The figure shows three views and two pictorial views of one solid part (mm, origin at its lowest corner). Answer the questions. A direction names the side the tool comes from. Coordinates: 2 decimals unless noted, no trailing zeros. Loops run counter-clockwise (first coordinate to the right, second up) from the corner with the lowest first, then second, coordinate; pieces in that order, holes last.
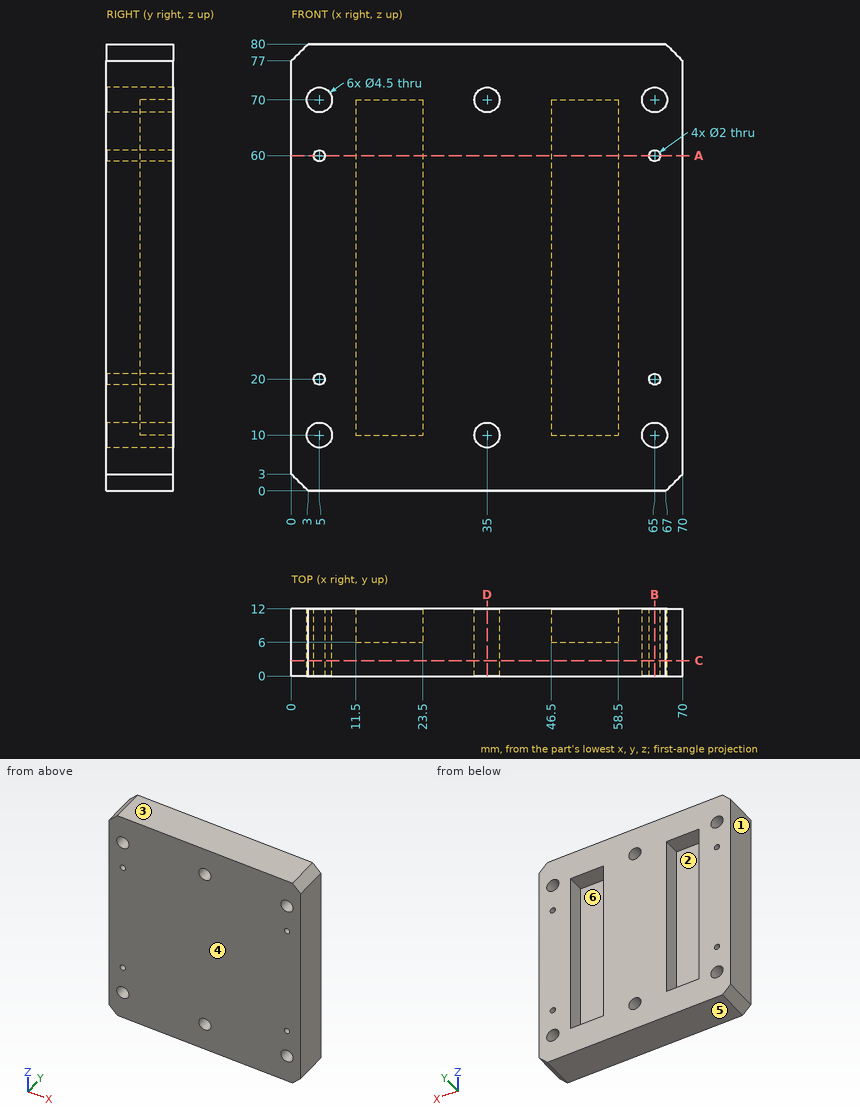
Q1. A cutting plane is placed at B-B (x = 65). Give the vertices of the cut face in (y, z), then the cut area to 3 significant figures.
Findings below:
outline: (0, 0) - (12, 0) - (12, 7.75) - (0, 7.75) - close; (0, 12.25) - (12, 12.25) - (12, 19) - (0, 19) - close; (0, 21) - (12, 21) - (12, 59) - (0, 59) - close; (0, 61) - (12, 61) - (12, 67.75) - (0, 67.75) - close; (0, 72.25) - (12, 72.25) - (12, 80) - (0, 80) - close
area: 804 mm2
Q2. A cutting plane is placed at C-C (y = 2.75). Count the separate pieces of the cut face and the enclosed holes in it, then the cut area to 3 significant figures.
Findings below:
separate pieces: 1
enclosed holes: 10
area: 5,470 mm2
Q3. Which of the six approach directions +Z, -Z, +X, -X, +Y, -Y give full straight-line access (tool end or side, diameter ignored) to the marked faces 1 and 2?
Findings below:
face 1: +Z, -Z, -X, +Y, -Y
face 2: +Y
Q4. Determine the mould class of the marked faces 3, 4, 5 and 6 for opening direction Z: +Z half, -Z half, draft (parallel to the pull), parting line (faces both ways), or undercut.
Findings below:
face 3: +Z half
face 4: draft
face 5: -Z half
face 6: undercut
Q5. A flat-ended cylindrical pin translates along its axis: pin 1 Ø1.5 at (x, z) = (54.5, 63.5) entering from +Y. Find the tip coordinate at first contact, or state that the pin passes through.
Findings below:
pin 1: stops at y = 6
Q6. Straight lines are drawn through the part: probe 1 along X at (y, z) = (11, 52.5); probe 2 along X at (y, z) = (8.25, 20); probe 3 along Z at (x, y) = (19, 9.5). For each, find the intervals that lie inside material, in ascending order.
Findings below:
probe 1: x = 0 to 11.5, 23.5 to 46.5, 58.5 to 70
probe 2: x = 0 to 4, 6 to 11.5, 23.5 to 46.5, 58.5 to 64, 66 to 70
probe 3: z = 0 to 10, 70 to 80
Q7. A cutting plane is placed at A-A (z = 60). Give the vertices of the cut face in (x, y), then the cut area to 3 significant figures.
Findings below:
outline: (0, 0) - (4, 0) - (4, 12) - (0, 12) - close; (6, 0) - (64, 0) - (64, 12) - (58.5, 12) - (58.5, 6) - (46.5, 6) - (46.5, 12) - (23.5, 12) - (23.5, 6) - (11.5, 6) - (11.5, 12) - (6, 12) - close; (66, 0) - (70, 0) - (70, 12) - (66, 12) - close
area: 648 mm2
Q8. A cutting plane is placed at D-D (x = 35). Give the vertices of the cut face in (y, z), then the cut area to 3 significant figures.
Findings below:
outline: (0, 0) - (12, 0) - (12, 7.75) - (0, 7.75) - close; (0, 12.25) - (12, 12.25) - (12, 67.75) - (0, 67.75) - close; (0, 72.25) - (12, 72.25) - (12, 80) - (0, 80) - close
area: 852 mm2
